Geometry: final body of the model. Coordinates: model frame, mm. Coordinates: 2 decimals unless noted, no trailing zeros. Order: outer loops, then holes, each group sorted by start corner. A loop starts at its lowest first (then second) coordinate and runs counter-clockwise, first axis right, second up. Notation, with made-up numbers: (41, 10.5) -> (62, 10.5) arc R33 cw to (62, 41.5) -> close; hole circle Ø10 at (15, 44.5). An arc over 180 degrees is marked (long way). Use CSV: the item, a comma, the result in double quotes. Start each with the question number.
from build123d import *

# Parameters (mm, degrees)
F2_ANGLE_BACK = 30
F2_ANGLE      = 60


with BuildPart() as f2:
    # F1 (on Front) → F2 (revolve)
    with BuildSketch(Plane.XZ, mode=Mode.PRIVATE) as f2_sk:
        with BuildLine():
            ThreePointArc((0, 140), (98.9949493661, 98.9949493661), (140, 0))
            Line((140, 0), (140, -30))
            Line((140, -30), (160, -30))
            Line((160, -30), (160, 0))
            ThreePointArc((160, 0), (113.1370849898, 113.1370849898), (0, 160))
            Line((0, 160), (0, 140))
        make_face()
    revolve(f2_sk.sketch.rotate(Axis((0, 0, 50), (0, 0, 1)), -F2_ANGLE_BACK), axis=Axis((0, 0, 50), (0, 0, 1)), revolution_arc=F2_ANGLE)


solid = f2.part
(1) First-contact query: pin 1 (1.5 mm diameter, centred on x = 108.5, y = 24, fed in from -Z); pin 2 (1 mm diameter, centred on y = -31, z = 99.5, fed in from -X); pin 3 (1.5 mm diameter, centred on x = 94.5, z = 92.5, fed in from +Y). Flat tips, straight axial feed; report the tip coordinate or a pass-through.
(2) Section C-C (x = 98.5). Return loops of the section in (y, z), then the cut area to 3 significant figures.
(3) Line query: line 1 (Y direction, x = 126.5, z = -13); line 2 (Z direction, x = 110.5, y = 20); line 3 (Z direction, x = 95.5, y = -21). Output: solid intervals per line, ascending. Write a range as from..to.
(4) Section D-D (y = -57.5). Return loops of the section in (x, z).
(5) Section A-A (y = 33). Return loops of the section in (x, z), then the cut area to 3 significant figures.
(6) Section B-B (z = 148). Return loops of the section in (x, y), then the cut area to 3 significant figures.
(7) Mould query, pull axis Y, two halves, no side actions, for faces 1 (the face through (159.996, -1.173, -14.79)), 2 (the face through (94.62, 54.63, 93.59)), 3 (the face through (139.996, -1.026, -15.21)), 4 (the face through (94.62, -54.63, 93.59)). Classes: pulls with the +Y half, pulls with the -Y half, needs draft (parallel to the pull), parting line crosses it, or undercut.
Check sheet entries:
1,pin 1,"stops at z = 84.17"
1,pin 2,"stops at x = 92.92"
1,pin 3,"stops at y = 54.99"
2,outline,"(-56.87, 81.63) arc R99.49 cw to (56.87, 81.63) -> (56.87, 112.53) arc R126.09 ccw to (-56.87, 112.53) -> close"
2,area,"3,170 mm^2"
3,line 1,"y = -73.03..-59.98, 59.98..73.03"
3,line 2,"z = 83.6..113.97"
3,line 3,"z = 100.19..126.64"
4,outline,"(99.59, 79.84) arc R127.65 cw to (127.65, 0) -> (127.65, -30) -> (149.31, -30) -> (149.31, 0) arc R149.31 ccw to (99.59, 111.24) -> close"
5,outline,"(57.16, 123.47) arc R136.06 cw to (136.06, 0) -> (136.06, -30) -> (156.56, -30) -> (156.56, 0) arc R156.56 ccw to (57.16, 145.75) -> close"
5,area,"4,120 mm^2"
6,outline,"(0, 0) -> (52.65, -30.4) arc R60.79 ccw to (52.65, 30.4) -> close"
6,area,"1,940 mm^2"
7,face 1,"parting line crosses it"
7,face 2,"pulls with the +Y half"
7,face 3,"undercut"
7,face 4,"pulls with the -Y half"
